Autodesk Inventor part; units mm, degrees
ref_plane "YZ Plane" through (0, 0, 0) normal (1, 0, 0) x (0, 1, 0)
ref_plane "XZ Plane" through (0, 0, 0) normal (0, 1, 0) x (-1, 0, 0)
ref_plane "XY Plane" through (0, 0, 0) normal (0, 0, 1) x (1, 0, 0)
sketch "Sketch1" plane through (0, 0, 0) normal (0, 1, 0) x (-1, 0, 0)
  circle A0 centre (-17.9853, 31.5522) radius 1.6
  circle A1 centre (22.0147, 11.5522) radius 1.6
  circle A2 centre (62.0147, 11.5522) radius 1.6
  circle A3 centre (102.0147, 11.5522) radius 1.6
  circle A4 centre (-17.9853, -8.4478) radius 1.6
  circle A5 centre (2.0147, 11.5522) radius 1.6
  circle A6 centre (-57.9853, 11.5522) radius 1.6
  circle A7 centre (-97.9853, 11.5522) radius 1.6
  circle A8 centre (-77.9853, 11.5522) radius 1.6
  circle A9 centre (-37.9853, 11.5522) radius 1.6
  circle A10 centre (-17.9853, -28.4478) radius 1.6
  circle A11 centre (-17.9853, 11.5522) radius 1.6
  circle A12 centre (-17.9853, 51.5522) radius 1.6
  circle A13 centre (82.0147, 11.5522) radius 1.6
  circle A14 centre (42.0147, 11.5522) radius 1.6
  line L0 (-9.6933, -37.4479) -> (-9.6933, -0.9478)
  arc A15 (-4.6933, 4.0522) -> (-9.6933, -0.9478) centre (-4.6933, -0.9478) ccw
  line L1 (-4.6933, 4.0522) -> (108.2535, 4.0522)
  line L2 (-26.2773, 59.9411) -> (-26.2773, 24.0522)
  arc A16 (-31.2773, 19.0522) -> (-26.2773, 24.0522) centre (-31.2773, 24.0522) ccw
  line L3 (-31.2773, 19.0522) -> (-110.8172, 19.0522)
  line L4 (-110.8172, 4.0522) -> (-31.2773, 4.0522)
  arc A17 (-26.2773, -0.9478) -> (-31.2773, 4.0522) centre (-31.2773, -0.9478) ccw
  line L5 (-26.2773, -0.9478) -> (-26.2773, -36.8367)
  line L6 (108.2535, 19.0522) -> (-4.6933, 19.0522)
  arc A18 (-9.6933, 24.0522) -> (-4.6933, 19.0522) centre (-4.6933, 24.0522) ccw
  line L7 (-9.6933, 24.0522) -> (-9.6933, 60.5523)
  circle A19 centre (-17.9853, 51.5522) radius 8.292
  circle A20 centre (-17.9853, -28.4478) radius 8.292
  circle A21 centre (102.0147, 11.5522) radius 7.5
  circle A22 centre (-97.9853, 11.5522) radius 7.5
  circle A23 centre (102.0147, 11.5522) radius 0.75
  circle A24 centre (82.0147, 11.5522) radius 0.75
  circle A25 centre (62.0147, 11.5522) radius 0.75
  circle A26 centre (42.0147, 11.5522) radius 0.75
  circle A27 centre (22.0147, 11.5522) radius 0.75
  circle A28 centre (2.0147, 11.5522) radius 0.75
  circle A29 centre (-17.9853, 11.5522) radius 0.75
  circle A30 centre (-37.9853, 11.5522) radius 0.75
  circle A31 centre (-57.9853, 11.5522) radius 0.75
  circle A32 centre (-77.9853, 11.5522) radius 0.75
  circle A33 centre (-97.9853, 11.5522) radius 0.75
  circle A34 centre (-17.9853, 51.5522) radius 0.75
  circle A35 centre (-17.9853, 31.5522) radius 0.75
  circle A36 centre (-17.9853, -8.4478) radius 0.75
  circle A37 centre (-17.9853, -28.4478) radius 0.75
  point P0 (0, 0)
  point P1 (-0.7536, 11.5522)
  point P2 (102.0147, 4.0522)
  point P3 (102.0147, 19.0522)
  point P4 (-9.6933, 51.5522)
  point P5 (-26.2773, 51.5522)
  point P6 (-97.9853, 19.0522)
  point P7 (-97.9853, 4.0522)
  point P8 (-26.2773, -28.4478)
  point P9 (-9.6933, -28.4478)
  dimension "d0" = 1.5
  dimension "d3" = 20
  dimension "d8" = 1.5
  dimension "d9" = 1.5
  dimension "d10" = 1.5
  dimension "d11" = 1.5
extrude "Extrusion1" add sketch "Sketch1" along normal blind 4.8 contours A0 | A1 | A2 | A3 | A4 | A5 | A6 | A7 | A8 | A9 | A10 | A11 | A12 | A13 | A14 | A20 L5 A17 L4 A22 L3 A16 L2 A19 L7 A18 L6 A21 L1 A15 L0 | A20 | A21 | A22 | A19
sketch "Sketch3" plane through (0, 4.8, 0) normal (0, 1, 0) x (1, 0, 0)
  line L0 (-102.0147, -19.0522) -> (4.6933, -19.0522)
  arc A0 (9.6933, -24.0522) -> (4.6933, -19.0522) centre (4.6933, -24.0522) ccw
  line L1 (9.6933, -24.0522) -> (9.6933, -51.5522)
  arc A1 (9.6933, -51.5522) -> (26.2773, -51.5522) centre (17.9853, -51.5522) ccw
  line L2 (26.2773, -51.5522) -> (26.2773, -24.0522)
  arc A2 (31.2773, -19.0522) -> (26.2773, -24.0522) centre (31.2773, -24.0522) ccw
  line L3 (31.2773, -19.0522) -> (97.9853, -19.0522)
  arc A3 (97.9853, -19.0522) -> (97.9853, -4.0522) centre (97.9853, -11.5522) ccw
  line L4 (97.9853, -4.0522) -> (31.2773, -4.0522)
  arc A4 (26.2773, 0.9478) -> (31.2773, -4.0522) centre (31.2773, 0.9478) ccw
  line L5 (26.2773, 0.9478) -> (26.2773, 28.4478)
  arc A5 (26.2773, 28.4478) -> (9.6933, 28.4478) centre (17.9853, 28.4478) ccw
  line L6 (9.6933, 28.4478) -> (9.6933, 0.9478)
  arc A6 (4.6933, -4.0522) -> (9.6933, 0.9478) centre (4.6933, 0.9478) ccw
  line L7 (4.6933, -4.0522) -> (-102.0147, -4.0522)
  arc A7 (-102.0147, -4.0522) -> (-102.0147, -19.0522) centre (-102.0147, -11.5522) ccw
  circle A8 centre (17.9853, 28.4478) radius 0.75
  circle A9 centre (97.9853, -11.5522) radius 0.75
  circle A10 centre (17.9853, -51.5522) radius 0.75
  circle A11 centre (17.9853, -31.5522) radius 0.75
  circle A12 centre (17.9853, -11.5522) radius 0.75
  circle A13 centre (17.9853, 8.4478) radius 0.75
  circle A14 centre (37.9853, -11.5522) radius 0.75
  circle A15 centre (77.9853, -11.5522) radius 0.75
  circle A16 centre (57.9853, -11.5522) radius 0.75
  circle A17 centre (-42.0147, -11.5522) radius 0.75
  circle A18 centre (-2.0147, -11.5522) radius 0.75
  circle A19 centre (-22.0147, -11.5522) radius 0.75
  circle A20 centre (-82.0147, -11.5522) radius 0.75
  circle A21 centre (-62.0147, -11.5522) radius 0.75
  circle A22 centre (-102.0147, -11.5522) radius 0.75
  point P0 (0, 0)
hole "Hole1" at (-102.0147, 4.8, 11.5522) at (-82.0147, 4.8, 11.5522) at (-62.0147, 4.8, 11.5522) at (-42.0147, 4.8, 11.5522) at (-22.0147, 4.8, 11.5522) at (-2.0147, 4.8, 11.5522) at (17.9853, 4.8, -28.4478) at (17.9853, 4.8, -8.4478) at (17.9853, 4.8, 11.5522) at (17.9853, 4.8, 31.5522) at (37.9853, 4.8, 11.5522) at (17.9853, 4.8, 51.5522) at (57.9853, 4.8, 11.5522) at (77.9853, 4.8, 11.5522) at (97.9853, 4.8, 11.5522) direction (0, -1, 0) diameter 3 end through all countersink diameter 6 countersink angle 90
properties part number "usztywnienie"
Check sheet for the modelled part. Datum: model origin and axes. Units: mm. A direction names the side the tool comes from. Round coordinates to 2 decimals unless told otherwise and drop trailing zeros. Loops run counter-clockwise (first coordinate to the right, second up) from the corner with the lowest first, then second, coordinate; pieces in that order, holes last.
1. Scan lines: probe 1 along Z at (x, y) = (32, 3.4); probe 2 along X at (y, z) = (3.6, 51.5); probe 3 along X at (y, z) = (0.55, -1.5). Record each from-to range of solid material in increasing order.
2. Gauge pin test, flat ends, axial feed: pin 1 Ø2.5 at (x, z) = (-42.01, 11.55) entering from +Y; pin 2 Ø2.5 at (x, y) = (-74, 2.5) entering from +Z; pin 3 Ø4 at (x, z) = (17.99, -8.45) entering from +Y; pin 4 Ø1 at (x, y) = (64.5, 3) entering from -Z. Record the tip position at first contact, or that the pin passes through.
3. Sectioned sample at A-A on x = 45.5. Record the boundary of the cut face in (y, z), and give its area (3 significant figures).
4. Set-up check for faces 1 (the flat face through (-49, 2, 19.052)), 2 (the cylindrical face through (18.168, 2.366, 59.842)), 3 (the flat face through (9.693, 2, -15)): record each of +Z, -Z, +X, -X, +Y, -Y from which the full face is reachable in a straight line by a thin tool's end or side.
5. Sectioned sample at C-C on z = -22. Record the boundary of the cut face in (x, y), and give its area (3 significant figures).
6. Sectioned sample at B-B on y = 2.55. Give the number of separate pieces and of enclosed holes in the cut face, and give its area (3 significant figures).
Recorded:
1. probe 1: z = 4.05 to 19.05
1. probe 2: x = 9.69 to 16.19, 19.78 to 26.28
1. probe 3: x = 9.69 to 26.28
2. pin 1: passes through
2. pin 2: stops at z = 19.05
2. pin 3: stops at y = 3.81
2. pin 4: stops at z = 4.05
3. outline: (0, 4.05) - (4.8, 4.05) - (4.8, 19.05) - (0, 19.05) - close
3. area: 72.0 mm2
4. face 1: +Z, -X, +Y, -Y
4. face 2: +Z, +Y, -Y
4. face 3: -Z, -X, +Y, -Y
5. outline: (9.69, 0) - (26.28, 0) - (26.28, 4.8) - (9.69, 4.8) - close
5. area: 79.6 mm2
6. separate pieces: 1
6. enclosed holes: 15
6. area: 4,390 mm2
